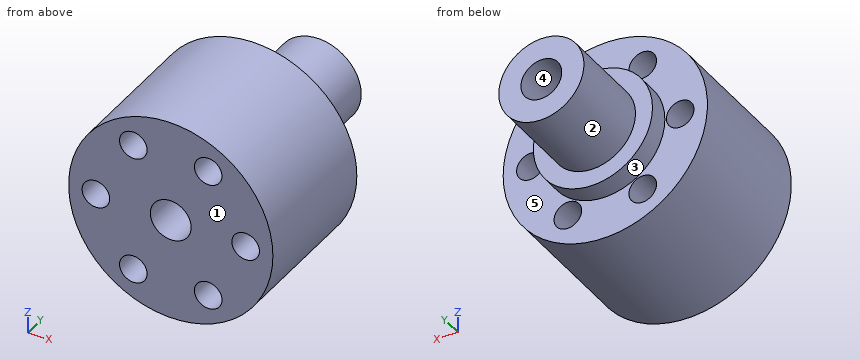
Autodesk Inventor part; units mm, degrees
ref_plane "YZ Plane" through (0, 0, 0) normal (1, 0, 0) x (0, 1, 0)
ref_plane "XZ Plane" through (0, 0, 0) normal (0, 1, 0) x (-1, 0, 0)
ref_plane "XY Plane" through (0, 0, 0) normal (0, 0, 1) x (1, 0, 0)
sketch "Sketch1" plane through (0, 0, 0) normal (0, 1, 0) x (-1, 0, 0)
  circle A0 centre (0, 0) radius 17.5
  dimension "d0" = 35
extrude "Extrusion1" add sketch "Sketch1" along normal blind 6
sketch "Sketch2" plane through (0, 6, 0) normal (0, 1, 0) x (1, 0, 0)
  circle A0 centre (0, 0) radius 12.5
  dimension "d3" = 25
extrude "Extrusion2" add sketch "Sketch2" along normal blind 25
sketch "Sketch3" plane through (0, 31, 0) normal (0, 1, 0) x (1, 0, 0)
  circle A0 centre (0, 0) radius 6
extrude "Extrusion3" cut sketch "Sketch3" against normal blind 100
sketch "Sketch4" plane through (0, 0, 0) normal (0, -1, 0) x (1, 0, 0)
  circle A0 centre (0, 0) radius 6
  circle A1 centre (0, 0) radius 30
  circle A2 centre (22, 0) radius 4.05
  circle A3 centre (11, 19.0526) radius 4.05
  circle A4 centre (-11, 19.0526) radius 4.05
  circle A5 centre (-22, 0) radius 4.05
  circle A6 centre (-11, -19.0526) radius 4.05
  circle A7 centre (11, -19.0526) radius 4.05
  dimension "d8" = 60
  dimension "d11" = 12
  dimension "d12" = 22
  dimension "d13" = 8.1
  dimension "d16" = 360
extrude "Extrusion4" add sketch "Sketch4" along normal blind 24
sketch "Sketch5" plane through (0, -24, 0) normal (0, -1, 0) x (1, 0, 0)
  circle A0 centre (0, 0) radius 30
  circle A1 centre (11, -19.0526) radius 4.05
  circle A2 centre (-11, -19.0526) radius 4.05
  circle A3 centre (-22, 0) radius 4.05
  circle A4 centre (-11, 19.0526) radius 4.05
  circle A5 centre (11, 19.0526) radius 4.05
  circle A6 centre (22, 0) radius 4.05
  circle A7 centre (0, 0) radius 6
extrude "Extrusion5" add sketch "Sketch5" along normal blind 16.7
properties part number "MiniPodsipnikNatag"
CAD build for the part. Positions are in the model's coordinates, mm. Face numbers are marked on the shaded views. A direction names the side the tool comes from. Give positions to 0.01 mm unless a question says otherwise; leave off trailing zeros. Loops run counter-clockwise (first coordinate to the right, second up) from the corner with the lowest first, then second, coordinate; pieces in that order, holes last. Notation, with made-up numbers: M 42,59.5 L 74,59.5 A28 ccw 74,97.5 Z; hole C -37.5,81.25 d8. An arc over 180 degrees is marked long. Write each question's results on one line, items separated by ' | '.
Q1. Band-saw the part on D-D on y = 1. Write the cut outline in (x, z), and give its area (3 significant figures).
Geometry check:
outline: C 0,0 d35; hole C 0,0 d12 | area: 849 mm²
Q2. Which spindle directions (+Z, -Z, +X, -X, +Y, -Y) get a long thin tool onto all of the face, cutting with end or side? Do the marked faces 1 and 2. Say none if no direction does.
Geometry check:
face 1: +Z, -Z, +X, -X, -Y | face 2: +Y
Q3. Band-saw the part on A-A on x = 0. Write the cut outline in (y, z).
Geometry check:
outline: M -40.7,-30 L 0,-30 L 0,-17.5 L 6,-17.5 L 6,-12.5 L 31,-12.5 L 31,-6 L -40.7,-6 Z; M -40.7,6 L 31,6 L 31,12.5 L 6,12.5 L 6,17.5 L 0,17.5 L 0,30 L -40.7,30 Z
Q4. Flat gauge pins, fed straight in: P1, Ø6.5, axis at x = 11, z = -19.05, coming from the +Y side; P2, Ø8, axis at x = -12.5, y = 2, coming from the -Z side; P3, Ø5, axis at x = -16, z = -21, coming from the +Y side; P4, Ø5, axis at y = 0, z = 7, coming from the +X side. Where does each tip first touch, or does it go through?
Geometry check:
P1: passes through | P2: stops at z = -28.61 | P3: stops at y = 0 | P4: stops at x = 29.66
Q5. Mould opens along X. For the marked faces 3, 4 and 5 say: pulls with the +X half, pulls with the -X half, needs draft (parallel to the pull), parting line crosses it, or undercut.
Geometry check:
face 3: parting line crosses it | face 4: undercut | face 5: needs draft
Q6. Band-saw the part on C-C on x = -11. Write the cut outline in (y, z), and give its area (3 significant figures).
Geometry check:
outline: M -40.7,-27.91 L 0,-27.91 L 0,-23.1 L -40.7,-23.1 Z; M -40.7,-15 L 0,-15 L 0,-13.61 L 6,-13.61 L 6,-5.94 L 31,-5.94 L 31,5.94 L 6,5.94 L 6,13.61 L 0,13.61 L 0,15 L -40.7,15 Z; M -40.7,23.1 L 0,23.1 L 0,27.91 L -40.7,27.91 Z | area: 2,070 mm²
Q7. Band-saw the part on B-B on z = 0. Write the cut outline in (x, y).
Geometry check:
outline: M -30,-40.7 L -26.05,-40.7 L -26.05,0 L -30,0 Z; M -17.95,-40.7 L -6,-40.7 L -6,31 L -12.5,31 L -12.5,6 L -17.5,6 L -17.5,0 L -17.95,0 Z; M 6,-40.7 L 17.95,-40.7 L 17.95,0 L 17.5,0 L 17.5,6 L 12.5,6 L 12.5,31 L 6,31 Z; M 26.05,-40.7 L 30,-40.7 L 30,0 L 26.05,0 Z
Q8. Probe probe 1 along Z at (x, y) = (-11, -19); probe 2 along Z at (x, y) = (0, -18); probe 3 along X at (y, z) = (-28.5, -1.5). List the from-to ranges inside material, lowest first.
Geometry check:
probe 1: z = -27.91 to -23.1, -15 to 15, 23.1 to 27.91 | probe 2: z = -30 to -6, 6 to 30 | probe 3: x = -29.96 to -25.76, -18.24 to -5.81, 5.81 to 18.24, 25.76 to 29.96
